Part model, mm, in its own coordinate system. Round coordinates to 2 decimals unless told otherwise and drop trailing zeros. Loops run counter-clockwise (first coordinate to the right, second up) from the corner with the lowest first, then second, coordinate; pieces in that order, holes last.
from build123d import *

# Parameters (mm, degrees)
SKETCH1_R               = 50.8
SKETCH1_R_2             = 49.2125
BOSS_EXTRUDE1_DEPTH     = 863.6
SKETCH2_W               = 6.35
SKETCH2_H               = 111.125
CUT_EXTRUDE1_DEPTH      = 51.8
CUT_EXTRUDE1_DEPTH_BACK = 51.8
SKETCH3_W               = 111.125
SKETCH3_H               = 6.35
CUT_EXTRUDE2_DEPTH      = 51.8
CUT_EXTRUDE2_DEPTH_BACK = 51.8


with BuildPart() as part:
    # Sketch1 → Boss-Extrude1 (new body)
    with BuildSketch(Plane.XY):
        Circle(SKETCH1_R)
        Circle(SKETCH1_R_2, mode=Mode.SUBTRACT)
    extrude(amount=BOSS_EXTRUDE1_DEPTH)

    # Sketch2 → Cut-Extrude1 (cut, two sides)
    with BuildSketch(Plane(origin=(0, 0, 0), x_dir=(1, 0, 0), z_dir=(0, 1, 0))) as cut_extrude1_sk:
        with Locations((0, -808.0375)):
            Rectangle(SKETCH2_W, SKETCH2_H)
    extrude(amount=CUT_EXTRUDE1_DEPTH, mode=Mode.SUBTRACT)
    extrude(cut_extrude1_sk.sketch, amount=-CUT_EXTRUDE1_DEPTH_BACK, mode=Mode.SUBTRACT)

    # Sketch3 → Cut-Extrude2 (cut, two sides)
    with BuildSketch(Plane(origin=(0, 0, 0), x_dir=(0, 0, -1), z_dir=(1, 0, 0))) as cut_extrude2_sk:
        with Locations((-808.0375, 0)):
            Rectangle(SKETCH3_W, SKETCH3_H)
    extrude(amount=CUT_EXTRUDE2_DEPTH, mode=Mode.SUBTRACT)
    extrude(cut_extrude2_sk.sketch, amount=-CUT_EXTRUDE2_DEPTH_BACK, mode=Mode.SUBTRACT)


solid = part.part
1) Slice it at C-C, the plane z = 63.5. Give the cut face in (x, y) (1 decimal), then the cut area to 3 significant figures.
Values:
outline: circle Ø101.6 at (0, 0); hole circle Ø98.4 at (0, 0)
area: 499 mm2
2) Mould opens along X. For faces 1 (the face through (46.94, 14.78, 425.75)), 2 (the face through (48.454, 15.259, 425.755)), 3 (the face through (36, 34, 863.6)) say: released by +X, released by -X, zero draft, split by the parting line, or undercut.
Values:
face 1: undercut
face 2: split by the parting line
face 3: zero draft
3) Wall check: line 1 along X through (y, z) = (0, 309); line 2 along X through (y, z) = (9, 555). Give the ranges that are in metal, low to high.
Values:
line 1: x = -50.8 to -49.21, 49.21 to 50.8
line 2: x = -50 to -48.38, 48.38 to 50
4) Drop flat-ended pins along their axis: pin 1 Ø2 at (y, z) = (24.5, 238) entering from +X; pin 2 Ø5 at (y, z) = (-31, 318.5) entering from +X; pin 3 Ø5 at (y, z) = (-14.5, 512.5) entering from -X. Give the stop position or say it passes through.
Values:
pin 1: stops at x = 45.04
pin 2: stops at x = 42.05
pin 3: stops at x = -49.36
5) Slice it at A-A, the plane y = 10.5. Give the cut face in (x, z).
Values:
outline: (-49.7, 0) - (-48.08, 0) - (-48.08, 863.6) - (-49.7, 863.6) - close; (48.08, 0) - (49.7, 0) - (49.7, 863.6) - (48.08, 863.6) - close
6) Slice it at B-B, the plane x = -34.5. Give the cut face in (y, z).
Values:
outline: (-37.29, 0) - (-35.09, 0) - (-35.09, 863.6) - (-37.29, 863.6) - close; (35.09, 0) - (37.29, 0) - (37.29, 863.6) - (35.09, 863.6) - close
